Here's how the part is built. I have some questions about the finished solid (model axes, mm). Face numbers are marked on the shaded views. Coordinates: 2 decimals unless noted, no trailing zeros. Order: outer loops, then holes, each group sorted by start corner. A loop starts at its lowest first (then second) coordinate and runs counter-clockwise, first axis right, second up. Notation, with made-up numbers: (-3.5, 14.25) - (54.5, 14.25) arc R25 ccw to (54.5, 49.25) - close; hole circle Ø1 at (-0.75, 36). An arc over 180 degrees is marked (long way). Answer in a Markdown table with one row per item. Add a question column.
Item 1: I want a section at A-A (y = 12.5). Please give me the cut outline in (x, z), plus the area to 3 significant figures.
Item 2: I want a section at B-B (x = 0). Please give me the cut outline in (y, z).
Item 3: Will these pins go through, and if not, where does the flat tip stop? pin 1 Ø1 at (y, z) = (-24.5, 8) entering from +X; pin 2 Ø1.5 at (x, y) = (-23.5, 4.5) entering from -Z; pin 3 Ø5 at (x, z) = (-56, 1.5) entering from -Y.
Item 4: I want a section at D-D (y = 47.5). Please give me the cut outline in (x, z), plus the area to 3 significant figures.
Item 5: I want a section at C-C (y = -54). Please give me the cut outline in (x, z), plus the area to 3 significant figures.
Item 6: If I drill on line 1 along Y through (x, z) = (80.5, 8.75); line 2 along Y through (x, z) = (-92, 6); line 3 along X through (y, z) = (77, 4.25), over which ranges is the centre line in solid material (lowest first)? Write a range as from..to.
Item 7: Thinking about a two-plate mould opening in X: for the marked faces 1 and 2, which applies, +X half, -X half, draft (parallel to the pull), parting line (faces both ways), or undercut?
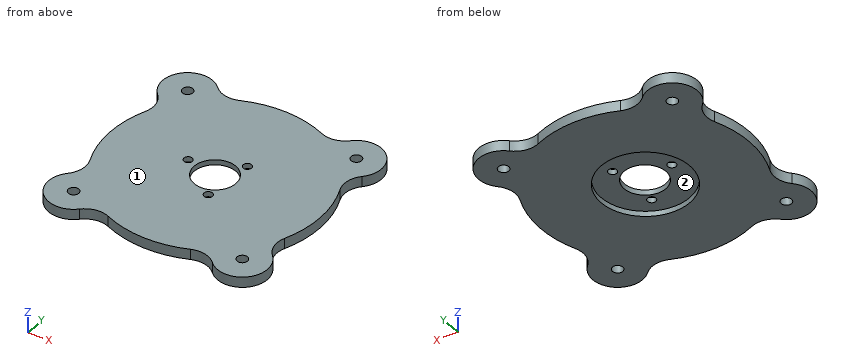
```python
from build123d import *

# Parameters (mm, degrees)
SKETCH1_R               = 5
SKETCH1_R_2             = 4
BOSS_EXTRUDE1_DEPTH     = 10
SKETCH3_R               = 20
CUT_EXTRUDE4_DEPTH      = 11
CUT_EXTRUDE4_DEPTH_BACK = 1
SKETCH6_R               = 42.5
CUT_EXTRUDE5_DEPTH      = 5


with BuildPart() as part:
    # Sketch1 → Boss-Extrude1 (new body)
    with BuildSketch(Plane.XY):
        with BuildLine():
            ThreePointArc((62.932503526, 96.873629023), (51.59941337, 90.83800352), (38.827006486, 92.154563465))
            ThreePointArc((38.827006486, 92.154563465), (0, 100), (-38.827006486, 92.154563465))
            ThreePointArc((-38.827006486, 92.154563465), (-51.59941337, 90.83800352), (-62.932503526, 96.873629023))
            ThreePointArc((-62.932503526, 96.873629023), (-96.873629023, 96.873629023), (-96.873629023, 62.932503526))
            ThreePointArc((-96.873629023, 62.932503526), (-90.83800352, 51.59941337), (-92.154563465, 38.827006486))
            ThreePointArc((-92.154563465, 38.827006486), (-100, 0), (-92.154563465, -38.827006486))
            ThreePointArc((-92.154563465, -38.827006486), (-90.83800352, -51.59941337), (-96.873629023, -62.932503526))
            ThreePointArc((-96.873629023, -62.932503526), (-96.873629023, -96.873629023), (-62.932503526, -96.873629023))
            ThreePointArc((-62.932503526, -96.873629023), (-51.59941337, -90.83800352), (-38.827006486, -92.154563465))
            ThreePointArc((-38.827006486, -92.154563465), (0, -100), (38.827006486, -92.154563465))
            ThreePointArc((38.827006486, -92.154563465), (51.59941337, -90.83800352), (62.932503526, -96.873629023))
            ThreePointArc((62.932503526, -96.873629023), (96.873629023, -96.873629023), (96.873629023, -62.932503526))
            ThreePointArc((96.873629023, -62.932503526), (90.83800352, -51.59941337), (92.154563465, -38.827006486))
            ThreePointArc((92.154563465, -38.827006486), (100, 0), (92.154563465, 38.827006486))
            ThreePointArc((92.154563465, 38.827006486), (90.83800352, 51.59941337), (96.873629023, 62.932503526))
            ThreePointArc((96.873629023, 62.932503526), (96.873629023, 96.873629023), (62.932503526, 96.873629023))
        make_face()
        with Locations((-79.903066991, 79.903065557)):
            Circle(SKETCH1_R, mode=Mode.SUBTRACT)
        with Locations((-79.903066274, -79.903067707)):
            Circle(SKETCH1_R, mode=Mode.SUBTRACT)
        with Locations((79.903066274, 79.903066274)):
            Circle(SKETCH1_R, mode=Mode.SUBTRACT)
        with Locations((79.903066991, -79.903066991)):
            Circle(SKETCH1_R, mode=Mode.SUBTRACT)
        with Locations((-28.659563911, 4.801920664)):
            Circle(SKETCH1_R_2, mode=Mode.SUBTRACT)
        with Locations((10.214266366, -24.539516671)):
            Circle(SKETCH1_R_2, mode=Mode.SUBTRACT)
        with Locations((14.823001416, 23.464491412)):
            Circle(SKETCH1_R_2, mode=Mode.SUBTRACT)
    extrude(amount=BOSS_EXTRUDE1_DEPTH)

    # Sketch3 → Cut-Extrude4 (cut, two sides)
    with BuildSketch(Plane.XY) as cut_extrude4_sk:
        Circle(SKETCH3_R)
    extrude(amount=CUT_EXTRUDE4_DEPTH, mode=Mode.SUBTRACT)
    extrude(cut_extrude4_sk.sketch, amount=-CUT_EXTRUDE4_DEPTH_BACK, mode=Mode.SUBTRACT)

    # Sketch6 → Cut-Extrude5 (cut)
    with BuildSketch(Plane.XY):
        with Locations((-0.919801826, 0.750296012)):
            Circle(SKETCH6_R)
    extrude(amount=CUT_EXTRUDE5_DEPTH, mode=Mode.SUBTRACT)


solid = part.part
```
Values follow:
| question | item | result |
|---|---|---|
| 1 | outline | (-99.22, 0) - (-41.76, 0) - (-41.76, 5) - (-15.61, 5) - (-15.61, 10) - (-99.22, 10) - close; (15.61, 5) - (39.92, 5) - (39.92, 0) - (99.22, 0) - (99.22, 10) - (15.61, 10) - close |
| 1 | area | 1,420 mm^2 |
| 2 | outline | (-100, 0) - (-41.74, 0) - (-41.74, 5) - (-20, 5) - (-20, 10) - (-100, 10) - close; (20, 5) - (43.24, 5) - (43.24, 0) - (100, 0) - (100, 10) - (20, 10) - close |
| 3 | pin 1 | stops at x = 97.08 |
| 3 | pin 2 | stops at z = 5 |
| 3 | pin 3 | stops at y = -93.45 |
| 4 | outline | (-90.43, 0) - (90.43, 0) - (90.43, 10) - (-90.43, 10) - close |
| 4 | area | 1,810 mm^2 |
| 5 | outline | (-91.45, 0) - (91.45, 0) - (91.45, 10) - (-91.45, 10) - close |
| 5 | area | 1,830 mm^2 |
| 6 | line 1 | y = -103.9..-84.87, -74.94..74.94, 84.87..103.9 |
| 6 | line 2 | y = -100.63..-55.54, -39.2..39.2, 55.54..100.63 |
| 6 | line 3 | x = -103.73..-83.97, -75.83..75.83, 83.97..103.73 |
| 7 | face 1 | draft |
| 7 | face 2 | undercut |
